Here's how the part is built. I have some questions about the finished solid (model axes, mm). Round coordinates to 2 decimals unless told otherwise and drop trailing zeros. Loops run counter-clockwise (first coordinate to the right, second up) from the corner with the lowest first, then second, coordinate; pieces in that order, holes last. Notation, with made-up numbers: M -32,-6.5 L 3,-6.5 A33 ccw 3,32.5 Z; hole C 83,-36.5 d3. An arc over 180 degrees is marked long. Answer as a JSON object with one key per item and string values.
Autodesk Inventor part; units mm, degrees
ref_plane "YZ Plane" through (0, 0, 0) normal (1, 0, 0) x (0, 1, 0)
ref_plane "XZ Plane" through (0, 0, 0) normal (0, 1, 0) x (-1, 0, 0)
ref_plane "XY Plane" through (0, 0, 0) normal (0, 0, 1) x (1, 0, 0)
sketch "Sketch1" plane through (0, 0, 0) normal (0, 0, 1) x (1, 0, 0)
  circle A0 centre (0, 0) radius 127
  dimension "d2" = 254
extrude "Extrusion1" add sketch "Sketch1" against normal blind 6.35
sketch "Sketch2" plane through (0, 0, 0) normal (0, 0, 1) x (1, 0, 0)
  circle A0 centre (0, 0) radius 127
hole "Hole1" at (0, 0, 0) direction (0, 0, -1) diameter 6.858 end through all
sketch "Sketch3" plane through (0, 0, 0) normal (0, 0, 1) x (1, 0, 0)
  circle A0 centre (0, 0) radius 3.429
  circle A1 centre (0, 0) radius 127
  circle A2 centre (0, 0) radius 117.475 construction
  point P0 (0, 117.475)
  dimension "d11" = 234.95
hole "Hole2" at (0, 117.475, 0) direction (0, 0, -1) diameter 7.874 end through all
pattern_circular "Circular Pattern1" count 16 over 360 about axis through (0, 0, 0) along (0, 0, -1) of "Hole2"
properties part number "GE-13036" material "Polyethylene, High Density"
Item 1: If we mould it in two halves opening along Y, with no side actions, what happens to faces 1 (the face through (-27.53, -123.98, -3.13)), 2 (the face through (-110.502, 48.365, -3.219)), 3 (the face through (-2, -26, -6.35))? For each: pulls with the +Y half, pulls with the -Y half, needs draft (parallel to the pull), parting line crosses it, or undercut.
Resolved:
{"face 1": "parting line crosses it", "face 2": "undercut", "face 3": "needs draft"}
Item 2: Please list where these lines run through material, in increasing order: probe 1 along X at (y, z) = (-110, -3.5); probe 2 along Y at (x, z) = (1.5, -1.5); probe 3 along X at (y, z) = (107, -4). Write a range as from..to.
Resolved:
{"probe 1": "-63.47..-48.61, -41.3..41.3, 48.61..63.47", "probe 2": "-126.99..-121.12, -113.83..-3.08, 3.08..113.83, 121.12..126.99", "probe 3": "-68.41..-48.58, -41.33..41.33, 48.58..68.41"}
Item 3: I want a section at D-D, the plane x = 73.5. Please give me the cut outline in (y, z).
Resolved:
{"outline": "M -103.57,-6.35 L 103.57,-6.35 L 103.57,0 L -103.57,0 Z"}
Item 4: I'm going to push flat-ended pins straight in: pin 1 Ø1 at (x, z) = (52.5, -1.5) entering from -Y; pin 2 Ø2 at (y, z) = (-40, -3.5) entering from -X; pin 3 Ø2 at (y, z) = (26.5, -5.5) entering from -X. Where does each tip first touch, or does it pass through?
Resolved:
{"pin 1": "y = -115.87", "pin 2": "x = -120.86", "pin 3": "x = -124.41"}
Item 5: I want a section at A-A, the plane x = 0. Please give me the cut outline in (y, z), then the cut area to 3 significant figures.
Resolved:
{"outline": "M -127,-6.35 L -121.41,-6.35 L -121.41,0 L -127,0 Z; M -113.54,-6.35 L -3.43,-6.35 L -3.43,0 L -113.54,0 Z; M 3.43,-6.35 L 113.54,-6.35 L 113.54,0 L 3.43,0 Z; M 121.41,-6.35 L 127,-6.35 L 127,0 L 121.41,0 Z", "area": "1,470 mm²"}
Item 6: I want a section at C-C, the plane z = -2. State how many separate pieces and enclosed holes the cut face has, then the cut area to 3 significant figures.
Resolved:
{"separate pieces": "1", "enclosed holes": "17", "area": "49,900 mm²"}
